Source: CAD feature listing. Evaluate the final solid. Frame: model axes, mm. Face numbers are marked on the shaded views. A direction names the side the tool comes from. Round coordinates to 2 decimals unless told otherwise and drop trailing zeros. Write each loop counter-clockwise with the first axis right and the second up, starting at its lowest first coordinate (ties: lowest second). Pieces come first, ordered by that corner, then holes. Notation, with made-up numbers: M -8.5,45.25 L 33.5,45.25 A23 cw 33.5,82.25 Z; hole C 3.25,-23 d7. An arc over 180 degrees is marked long. Answer in a Markdown table with one row per item. Add a question column.
Item 1: Contact query for flat-ended pins moving along their axis: pin 1 (2 mm diameter, centred on x = 0, y = -7.5, fed in from +Z); pin 2 (1.6 mm diameter, centred on y = 8, z = 1, fed in from +X); pin 3 (2 mm diameter, centred on x = -5.5, y = -0.5, fed in from -Z). Output: stop coordinate, or through.
Item 2: Set-up query: the marked faces 1, 2, 3 and 4. Return all of +Z, -Z, +X, -X, +Y, -Y with unobstructed straight access to the full face (end or side cutting, diameter ignored); none if empty.
Item 3: Cut plane A-A on z = 0.5. Return loops of the section in (x, y), and give its area (3 significant figures).
Item 4: Cut plane B-B on y = 6. Return loops of the section in (x, z).
Item 5: Material intervals for probe 1 along X at (y, z) = (-7.25, 1); probe 2 along Z at (x, y) = (5.75, 0.5), sorted ascending.
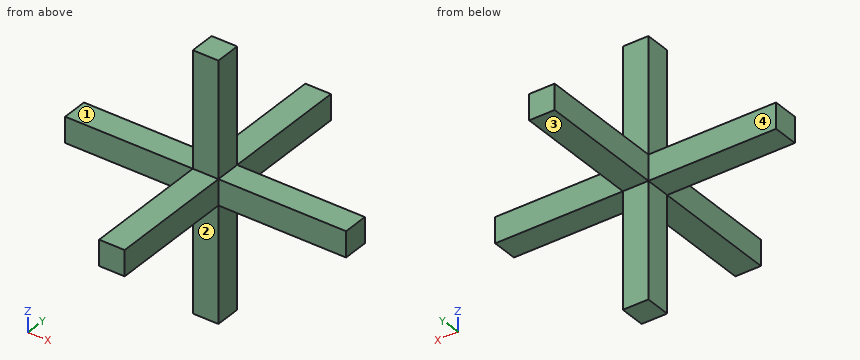
from build123d import *

# Parameters (mm, degrees)
PAD_DEPTH    = 2
SKETCH001_W  = 2
SKETCH001_H  = 2
PAD001_DEPTH = 9
SKETCH002_W  = 2
SKETCH002_H  = 2
PAD002_DEPTH = 9


with BuildPart() as part:
    # Sketch → Pad (new body)
    with BuildSketch(Plane.XY):
        Polygon((-1, 1), (-1, 11), (1, 11), (1, 1), (11, 1), (11, -1), (1, -1), (1, -11), (-1, -11), (-1, -1), (-11, -1), (-11, 1), align=None)
    extrude(amount=PAD_DEPTH)

    # Sketch001 → Pad001 (new body)
    with BuildSketch(Plane.XY.offset(2)):
        Rectangle(SKETCH001_W, SKETCH001_H)
    extrude(amount=PAD001_DEPTH)

    # Sketch002 → Pad002 (new body)
    with BuildSketch(Plane(origin=(0, 0, 0), x_dir=(1, 0, 0), z_dir=(0, 0, -1))):
        Rectangle(SKETCH002_W, SKETCH002_H)
    extrude(amount=PAD002_DEPTH)


solid = part.part
Results below:
| question | item | result |
|---|---|---|
| 1 | pin 1 | z = 2 |
| 1 | pin 2 | x = 1 |
| 1 | pin 3 | z = 0 |
| 2 | face 1 | +Z, -X, +Y, -Y |
| 2 | face 2 | -Z, +X, -X, -Y |
| 2 | face 3 | -Z, +X, -X, +Y |
| 2 | face 4 | +Z, -Z, -X, +Y |
| 3 | outline | M -11,-1 L -1,-1 L -1,-11 L 1,-11 L 1,-1 L 11,-1 L 11,1 L 1,1 L 1,11 L -1,11 L -1,1 L -11,1 Z |
| 3 | area | 84.0 mm2 |
| 4 | outline | M -1,0 L 1,0 L 1,2 L -1,2 Z |
| 5 | probe 1 | -1 to 1 |
| 5 | probe 2 | 0 to 2 |
